Geometry check sheet. Reference: the model listing, model coordinates, mm. Coordinates: 2 decimals unless noted, no trailing zeros. Order: outer loops, then holes, each group sorted by start corner. A loop starts at its lowest first (then second) coordinate and runs counter-clockwise, first axis right, second up.
```python
from build123d import *

# Parameters (mm, degrees)
SKETCH_3_R          = 2.5
CUT_EXTRUDE_1_DEPTH = 0.2
CUT_EXTRUDE_2_DEPTH = 0.2
CUT_EXTRUDE_START   = -0.2
SKETCH_5_R          = 2.5
CUT_EXTRUDE_3_DEPTH = 0.2
SKETCH_7_R          = 0.3
EXTRUDE_2_DEPTH     = 5.2


with BuildPart() as part:
    # Эскиз2 → Повернуть1 (revolve)
    with BuildSketch(Plane.XY):
        with BuildLine():
            Line((0, 0), (3.5, 0))
            ThreePointArc((3.5, 0), (3.853553391, 0.146446609), (4, 0.5))
            ThreePointArc((4, 0.5), (3.964238345, 0.685695338), (3.862068966, 0.844827586))
            ThreePointArc((3.862068966, 0.844827586), (3.5, 1.75), (3.862068966, 2.655172414))
            ThreePointArc((3.862068966, 2.655172414), (3.964238345, 2.814304662), (4, 3))
            Line((4, 3), (4, 11.5))
            ThreePointArc((4, 11.5), (3.853553391, 11.853553391), (3.5, 12))
            Line((3.5, 12), (0, 12))
            Line((0, 12), (0, 0))
        make_face()
    revolve(axis=Axis((0, 0, 0), (0, 1, 0)))

    # Эскиз3 → Вырез-Вытянуть1 (cut)
    with BuildSketch(Plane(origin=(0, 12, 0), x_dir=(1, 0, 0), z_dir=(0, 1, 0))):
        with Locations(Location((0, 0, 0), (0, 0, 180))):
            Circle(SKETCH_3_R)
    extrude(amount=-CUT_EXTRUDE_1_DEPTH, mode=Mode.SUBTRACT)

    # Эскиз4 → Вырез-Вытянуть2 (cut)
    with BuildSketch(Plane(origin=(0, 11.8, 0), x_dir=(1, 0, 0), z_dir=(0, 1, 0))):
        with BuildLine():
            Line((-0.25, -0.25), (-0.25, -2))
            ThreePointArc((-0.25, -2), (-0.179705627, -2.169705627), (-0.01, -2.24))
            Line((-0.01, -2.24), (0.01, -2.24))
            ThreePointArc((0.01, -2.24), (0.179705627, -2.169705627), (0.25, -2))
            Line((0.25, -2), (0.25, -0.25))
            Line((0.25, -0.25), (2, -0.25))
            ThreePointArc((2, -0.25), (2.169705627, -0.179705627), (2.24, -0.01))
            Line((2.24, -0.01), (2.24, 0.01))
            ThreePointArc((2.24, 0.01), (2.169705627, 0.179705627), (2, 0.25))
            Line((2, 0.25), (0.25, 0.25))
            Line((0.25, 0.25), (0.25, 2))
            ThreePointArc((0.25, 2), (0.179705627, 2.169705627), (0.01, 2.24))
            Line((0.01, 2.24), (-0.01, 2.24))
            ThreePointArc((-0.01, 2.24), (-0.179705627, 2.169705627), (-0.25, 2))
            Line((-0.25, 2), (-0.25, 0.25))
            Line((-0.25, 0.25), (-2, 0.25))
            ThreePointArc((-2, 0.25), (-2.169705627, 0.179705627), (-2.24, 0.01))
            Line((-2.24, 0.01), (-2.24, -0.01))
            ThreePointArc((-2.24, -0.01), (-2.169705627, -0.179705627), (-2, -0.25))
            Line((-2, -0.25), (-0.25, -0.25))
        make_face()
    extrude(amount=-CUT_EXTRUDE_2_DEPTH, mode=Mode.SUBTRACT)

    # Эскиз5 → Вырез-Вытянуть3 (cut)
    with BuildSketch(Plane.XZ.offset(CUT_EXTRUDE_START)):
        with Locations(Location((0, 0, 0), (0, 0, 180))):
            Circle(SKETCH_5_R)
    extrude(amount=CUT_EXTRUDE_3_DEPTH, mode=Mode.SUBTRACT)

    # Эскиз7 → Бобышка-Вытянуть2 (add)
    with BuildSketch(Plane.XZ.offset(-0.2)):
        with Locations((-1.75, 0)):
            Circle(SKETCH_7_R)
        with Locations((1.75, 0)):
            Circle(SKETCH_7_R)
    extrude(amount=EXTRUDE_2_DEPTH)


solid = part.part
```
Item 1: Depth check by flat-ended pin: P1, Ø3, axis at x = 0, z = 0, coming from the +Y side; P2, Ø1, axis at y = 2, z = 3, coming from the -X side. Enter the tip coordinate at first touch or a pass-through.
Item 2: Release check for a two-part mould opening along X. For faces 1 (the face through (-0.867, 7.31, 3.905)), 2 (the face through (2, 12, 2)), 3 (the face through (0, 0.2, 0)) record: pulls with the +X half, pulls with the -X half, needs draft (parallel to the pull), parting line crosses it, or undercut.
Item 3: Sectioned sample at C-C (y = 1.5). Record the cut outline in (x, z).
Item 4: Sectioned sample at B-B (y = 10). Record the cut outline in (x, z), and give its area (3 significant figures).
Item 5: Sectioned sample at A-A (y = -3). Record the cut outline in (x, z), and give its area (3 significant figures).
Item 6: Thickness scan on line 1 along Y through (x, z) = (3.25, 1); line 2 along Y through (x, z) = (-1.75, -0.5); line 3 along Z through (x, y) = (0, 11.9). Record the ranges inside material, lowest first.
Geometry check:
1. P1: stops at y = 11.8
1. P2: stops at x = -2.52
2. face 1: parting line crosses it
2. face 2: needs draft
2. face 3: undercut
3. outline: circle Ø7.05 at (0, 0)
4. outline: circle Ø8 at (0, 0)
4. area: 50.3 mm2
5. outline: circle Ø0.6 at (-1.75, 0); circle Ø0.6 at (1.75, 0)
5. area: 0.565 mm2
6. line 1: y = 0 to 12
6. line 2: y = 0.2 to 11.8
6. line 3: z = -3.8 to -2.5, 2.5 to 3.8
